from build123d import *

# Parameters (mm, degrees)
BOSS_EXTRUDE1_DEPTH      = 2.4892
BOSS_EXTRUDE1_DEPTH_BACK = 2.4892
SKETCH1_R                = 7.9375
SKETCH1_R_2              = 3.175
FILLET1_R                = 0.254
SKETCH2_R                = 7.4295
SKETCH2_R_2              = 3.429
CUT_EXTRUDE1_DEPTH       = 0.254


with BuildPart() as part:
    # Sketch1 → Boss-Extrude1 (new, two sides: drawn at the far end of the back side and taken through both)
    with BuildSketch(Plane(origin=(0, 0, 0), x_dir=(1, 0, 0), z_dir=(0, 1, 0)).offset(-BOSS_EXTRUDE1_DEPTH_BACK)):
        with Locations(Location((0, 0, 0), (0, 0, 270))):
            Circle(SKETCH1_R)
        with Locations(Location((0, 0, 0), (0, 0, 270))):
            Circle(SKETCH1_R_2, mode=Mode.SUBTRACT)
    extrude(amount=BOSS_EXTRUDE1_DEPTH + BOSS_EXTRUDE1_DEPTH_BACK)

    # Fillet1
    fillet1_edges = [part.edges().sort_by_distance(p)[0] for p in [
        (0, -2.4892, -7.9375),
        (0, 2.4892, -7.9375),
    ]]
    fillet(fillet1_edges, radius=FILLET1_R)

    # Sketch2 → Cut-Extrude1 (cut)
    with BuildSketch(Plane(origin=(0, 2.4892, 0), x_dir=(1, 0, 0), z_dir=(0, 1, 0))):
        with Locations(Location((0, 0, 0), (0, 0, 270))):
            Circle(SKETCH2_R)
        with Locations(Location((0, 0, 0), (0, 0, 270))):
            Circle(SKETCH2_R_2, mode=Mode.SUBTRACT)
    cut_extrude1 = extrude(amount=-CUT_EXTRUDE1_DEPTH, mode=Mode.SUBTRACT)

    # Mirror1: Cut-Extrude1 across plane
    add(cut_extrude1.mirror(Plane.ZX), mode=Mode.SUBTRACT)


solid = part.part
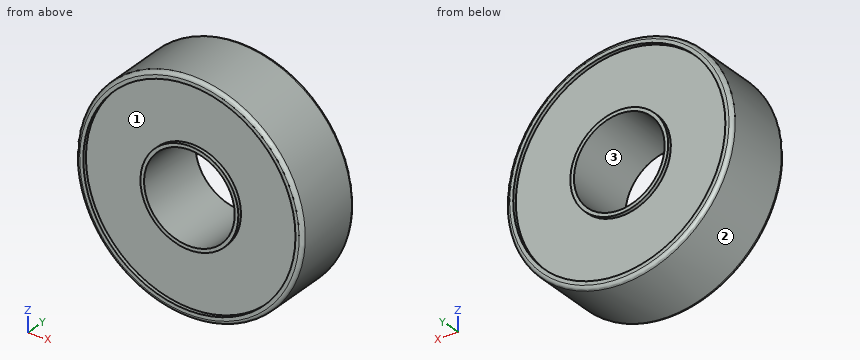
Here's how the part is built. I have some questions about the finished solid (model axes, mm). Face numbers are marked on the shaded views. Round coordinates to 2 decimals unless told otherwise and drop trailing zeros. One line per question, with ' | ' between items.
1) We'd pull the mould along Z, two halves only. Please class the marked faces 1, 2 and 3: released by +Z, released by -Z, zero draft, split by the parting line, or undercut.
Checked values:
face 1: undercut | face 2: split by the parting line | face 3: undercut
2) I need wall thicknesses on line 1 (X direction, y = 2.4, z = 0) (1 decimal); line 2 (Y direction, x = 7, z = -1); line 3 (X direction, y = 1.5, z = 0) (1 decimal). Which ranges of each line are inside material? Lowest first, please.
Checked values:
line 1: x = -7.9 to -7.4, -3.4 to -3.2, 3.2 to 3.4, 7.4 to 7.9 | line 2: y = -2.24 to 2.24 | line 3: x = -7.9 to -3.2, 3.2 to 7.9
3) I'm going to push a flat-ended pin straight in: pin 1 Ø1.5 at (y, z) = (1, 6) entering from -X. Where does the tip first touch, or does it pass through?
Checked values:
pin 1: stops at x = -5.95
